from build123d import *

# Parameters (mm, degrees)
SKETCH1_R                    = 37.5
BOSS_EXTRUDE1_DEPTH          = 9.6
CUT_EXTRUDE2_START           = -9.6
CUT_EXTRUDE2_DEPTH           = 9.6
SKETCH4_R                    = 45
SKETCH4_R_2                  = 37.5
BOSS_EXTRUDE2_DEPTH          = 9.6
BOSS_EXTRUDE3_START          = -8.6
BOSS_EXTRUDE3_DEPTH          = 8.6
SKETCH7_R                    = 2
CUT_EXTRUDE3_DEPTH           = 65.359614666
SKETCH14_R                   = 5
SKETCH14_R_2                 = 2
BOSS_EXTRUDE5_DEPTH          = 1.5
CHAMFER1_SIZE                = 1.5
CIRPATTERN2_COUNT            = 3
CHAMFER1_OF_CIRPATTERN2_SIZE = 1.5
BOSS_EXTRUDE4_START          = -9.6
BOSS_EXTRUDE4_DEPTH          = 9.6
FILLET1_R                    = 10
SKETCH12_R                   = 1.5
CUT_EXTRUDE6_DEPTH           = 66.773550915
LPATTERN1_COUNT              = 10
LPATTERN1_PITCH              = 10
CUT_EXTRUDE7_DEPTH           = 66.773550915
FILLET3_R                    = 1
CIRPATTERN3_COUNT            = 3
FILLET3_OF_CIRPATTERN3_R     = 1


# Read off the part's stored shape, not the designer's step: Cut-Extrude2
# Some blends are built 0.0001 mm under size
with BuildPart() as part:
    # Sketch1 → Boss-Extrude1 (new body)
    with BuildSketch(Plane(origin=(0, 0, 0), x_dir=(1, 0, 0), z_dir=(0, 1, 0))):
        with Locations(Location((0, 0, 0), (0, 0, 270))):
            Circle(SKETCH1_R)
    extrude(amount=BOSS_EXTRUDE1_DEPTH)

    # Cut-Extrude2 outline → Cut-Extrude2 (cut)
    with BuildSketch(Plane(origin=(0, 9.6, 0), x_dir=(1, 0, 0), z_dir=(0, 1, 0)).offset(CUT_EXTRUDE2_START)):
        with BuildLine():
            ThreePointArc((-24.104535363, -28.726666617), (0, -24.760936498), (24.104535363, -28.726666617))
            ThreePointArc((24.104535363, -28.726666617), (32.475952642, -18.75), (36.930290738, -6.511806663))
            ThreePointArc((36.930290738, -6.511806663), (21.443600029, 12.380468249), (12.825755375, 35.238473279))
            ThreePointArc((12.825755375, 35.238473279), (0, 37.5), (-12.825755375, 35.238473279))
            ThreePointArc((-12.825755375, 35.238473279), (-21.443600029, 12.380468249), (-36.930290738, -6.511806663))
            ThreePointArc((-36.930290738, -6.511806663), (-32.475952642, -18.75), (-24.104535363, -28.726666617))
        make_face()
    extrude(amount=CUT_EXTRUDE2_DEPTH, mode=Mode.SUBTRACT)

    # Sketch4 → Boss-Extrude2 (add)
    with BuildSketch(Plane(origin=(0, 0, 0), x_dir=(1, 0, 0), z_dir=(0, 1, 0))):
        with Locations(Location((0, 0, 0), (0, 0, 270))):
            Circle(SKETCH4_R)
        Circle(SKETCH4_R_2, mode=Mode.SUBTRACT)
    extrude(amount=BOSS_EXTRUDE2_DEPTH)

    # Sketch6 → Boss-Extrude3 (add)
    with BuildSketch(Plane(origin=(0, 9.6, 0), x_dir=(1, 0, 0), z_dir=(0, 1, 0)).offset(BOSS_EXTRUDE3_START)):
        with BuildLine():
            ThreePointArc((24.104535363, -28.726666617), (32.475952642, -18.75), (36.930290738, -6.511806663))
            ThreePointArc((36.930290738, -6.511806663), (21.443600029, 12.380468249), (12.825755375, 35.238473279))
            ThreePointArc((12.825755375, 35.238473279), (0, 37.5), (-12.825755375, 35.238473279))
            ThreePointArc((-12.825755375, 35.238473279), (-21.443600029, 12.380468249), (-36.930290738, -6.511806663))
            ThreePointArc((-36.930290738, -6.511806663), (-32.475952642, -18.75), (-24.104535363, -28.726666617))
            ThreePointArc((-24.104535363, -28.726666617), (0, -24.760936498), (24.104535363, -28.726666617))
        make_face()
    extrude(amount=BOSS_EXTRUDE3_DEPTH)

    # Sketch7 → Cut-Extrude3 (cut, through all)
    with BuildSketch(Plane(origin=(0, 9.6, 0), x_dir=(1, 0, 0), z_dir=(0, 1, 0))):
        with Locations(Location((0, 18, 0), (0, 0, 270))):
            Circle(SKETCH7_R)
    cut_extrude3 = extrude(amount=-CUT_EXTRUDE3_DEPTH, mode=Mode.SUBTRACT)

    # Sketch14 → Boss-Extrude5 (add)
    with BuildSketch(Plane.XZ.offset(-1)):
        with Locations(Location((0, -18, 0), (0, 0, 90))):
            Circle(SKETCH14_R)
        with Locations(Location((0, -18, 0), (0, 0, 90))):
            Circle(SKETCH14_R_2, mode=Mode.SUBTRACT)
    boss_extrude5 = extrude(amount=BOSS_EXTRUDE5_DEPTH)

    # Chamfer1
    chamfer1_edges = [part.edges().sort_by_distance(p)[0] for p in [
        (0, 1, -23),
    ]]
    chamfer(chamfer1_edges, length=CHAMFER1_SIZE - 0.0001)  # a hair under: the kernel refuses the full size

    # CirPattern2: Cut-Extrude3, Boss-Extrude5 ×3 about axis
    cirpattern2_axis = Axis((0, 0, 0), (0, 1, 0))
    add([cut_extrude3.rotate(cirpattern2_axis, i * 360 / CIRPATTERN2_COUNT) for i in range(1, CIRPATTERN2_COUNT)], mode=Mode.SUBTRACT)
    add([boss_extrude5.rotate(cirpattern2_axis, i * 360 / CIRPATTERN2_COUNT) for i in range(1, CIRPATTERN2_COUNT)])

    # Chamfer1 of CirPattern2
    chamfer1_of_cirpattern2_edges = [part.edges().sort_by_distance(p)[0] for p in [
        (-19.918584287, 1, 11.5),
        (19.918584287, 1, 11.5),
    ]]
    chamfer(chamfer1_of_cirpattern2_edges, length=CHAMFER1_OF_CIRPATTERN2_SIZE - 0.0001)  # a hair under: the kernel refuses the full size

    # Sketch11 → Boss-Extrude4 (add)
    with BuildSketch(Plane(origin=(0, 9.6, 0), x_dir=(1, 0, 0), z_dir=(0, 1, 0)).offset(BOSS_EXTRUDE4_START)):
        with BuildLine():
            ThreePointArc((-22.449944321, 39), (0, 45), (22.449944321, 39))
            Line((22.449944321, 39), (25, 39))
            Line((25, 39), (25, 47))
            Line((25, 47), (-25, 47))
            Line((-25, 47), (-25, 39))
            Line((-25, 39), (-22.449944321, 39))
        make_face()
    extrude(amount=BOSS_EXTRUDE4_DEPTH)

    # Fillet1
    # the kernel refuses this fillet: 10 mm, written as the material it adds along each edge
    with BuildSketch(Plane(origin=(-22.449944321, 0, -39), x_dir=(-1, 0, 0), z_dir=(0, 1, 0))) as fillet1_piece_1:
        with BuildLine():
            CenterArc((11.645047875, -4.157056285), FILLET1_R, 128.309485754, 27.126753117)
            ThreePointArc((5.445958385, 3.689681222), (2.79048981, 1.745195143), (0, 0))
            Line((0, 0), (2.550055679, 0))
        make_face()
    extrude(amount=9.6)
    with BuildSketch(Plane(origin=(22.449944321, 0, -39), x_dir=(1, 0, 0), z_dir=(0, 1, 0))) as fillet1_piece_2:
        with BuildLine():
            CenterArc((11.645047875, 4.157056285), FILLET1_R, 204.563761129, 27.126753117)
            ThreePointArc((5.445958385, -3.689681222), (2.79048981, -1.745195143), (0, 0))
            Line((0, 0), (2.550055679, 0))
        make_face()
    extrude(amount=9.6)

    # Sketch12 → Cut-Extrude6 (cut, through all)
    with BuildSketch(Plane.XZ):
        with Locations(Location((-20, -43, 0), (0, 0, 270))):
            Circle(SKETCH12_R)
    cut_extrude6 = extrude(amount=-CUT_EXTRUDE6_DEPTH, mode=Mode.SUBTRACT)

    # LPattern1: Cut-Extrude6 ×10
    with Locations(*[(i * LPATTERN1_PITCH, 0, 0) for i in range(1, LPATTERN1_COUNT)]):
        add(cut_extrude6, mode=Mode.SUBTRACT)

    # Sketch13 → Cut-Extrude7 (cut, through all)
    with BuildSketch(Plane.XZ):
        with BuildLine():
            ThreePointArc((-22.11228446, 33.332369792), (0, 29.760936498), (22.11228446, 33.332369792))
            ThreePointArc((22.11228446, 33.332369792), (0, 40), (-22.11228446, 33.332369792))
        make_face()
    cut_extrude7 = extrude(amount=-CUT_EXTRUDE7_DEPTH, mode=Mode.SUBTRACT)

    # Fillet3
    fillet3_edges = [part.edges().sort_by_distance(p)[0] for p in [
        (-22.11228446, 4.8, 33.332369792),
        (22.11228446, 4.8, 33.332369792),
    ]]
    fillet(fillet3_edges, radius=FILLET3_R)

    # CirPattern3: Cut-Extrude7 ×3 about axis
    cirpattern3_axis = Axis((0, 0, 0), (0, 1, 0))
    for i in range(1, CIRPATTERN3_COUNT):
        add(cut_extrude7.rotate(cirpattern3_axis, i * 360 / CIRPATTERN3_COUNT), mode=Mode.SUBTRACT)

    # Fillet3 of CirPattern3
    fillet3_of_cirpattern3_edges = [part.edges().sort_by_distance(p)[0] for p in [
        (39.922821238, 4.8, 2.483615182),
        (17.810536778, 4.8, -35.815984974),
        (-17.810536778, 4.8, -35.815984974),
        (-39.922821238, 4.8, 2.483615182),
    ]]
    fillet(fillet3_of_cirpattern3_edges, radius=FILLET3_OF_CIRPATTERN3_R)


solid = part.part
Design review of the part built by this model. Coordinates are the model's own, in mm. A direction names the side the tool comes from. Coordinates: 2 decimals unless noted, no trailing zeros. Order: outer loops, then holes, each group sorted by start corner. A loop starts at its lowest first (then second) coordinate and runs counter-clockwise, first axis right, second up. Notation, with made-up numbers: M -2.5,72 L 50.5,72 A15 cw 50.5,94 Z; hole C 10.25,-20.5 d8. An arc over 180 degrees is marked long. Use a Markdown table: item, result.
(1) For P1, Ø2, axis at y = 2, z = -23, coming from the +X side; P2, Ø2, axis at y = 6.5, z = 3.5, coming from the -X side; P3, Ø5, axis at x = 14.5, y = 2.5, coming from the +Z side, all flat-tipped, find the tip position at first contact; note any pin that passes through.
Worked answers:
| item | result |
|---|---|
| P1 | stops at x = 39.26 |
| P2 | stops at x = -44.93 |
| P3 | stops at z = 43.37 |
(2) For faces 1 (the cylindrical face through (32.384, 0.493, 18.908)), 2 (the cylindrical face through (-25.63, 4.73, -15.13)), 3 (the flat face through (2.2, -0.5, -18.1)), list the 3-axis set-ups (+Z, -Z, +X, -X, +Y, -Y) from which the entire face can be reached by the end or side of a thin tool; tool diameter is ignored.
Worked answers:
| item | result |
|---|---|
| face 1 | -Y |
| face 2 | +Y, -Y |
| face 3 | +Z, -Z, +X, -X, -Y |
(3) Add section C-C (z = 17.5). Give the boundary of the cut face in (x, y), then the cut area to 3 significant figures.
Worked answers:
| item | result |
|---|---|
| outline | M -41.46,0 L -33.17,0 L -33.17,1 L 33.17,1 L 33.17,0 L 41.46,0 L 41.46,9.6 L -41.46,9.6 Z |
| area | 730 mm2 |
(4) Wall thickness on probe 1 along X at (y, z) = (7.25, -43); probe 2 along Z at (x, y) = (-9, 0.5); probe 3 along X at (y, z) = (0.75, 7.5): over which ranges is each line inside the solid? List them lowest first.
Worked answers:
| item | result |
|---|---|
| probe 1 | x = -25 to -21.5, -18.5 to -11.5, -8.5 to -1.5, 1.5 to 8.5, 11.5 to 18.5, 21.5 to 25 |
| probe 2 | z = -47 to -44.12, -41.88 to -36.4, 25.3 to 30.34, 38.97 to 44.09 |
| probe 3 | x = -44.37 to -36.74, -21.66 to -16.91, -14.27 to -9.52, 9.52 to 14.27, 16.91 to 21.66, 36.74 to 44.37 |
(5) Add section A-A (x = -34). Give the boundary of the cut face in (y, z), then the cut area to 3 significant figures.
Worked answers:
| item | result |
|---|---|
| outline | M 0,-29.48 L 9.6,-29.48 L 9.6,-21.07 L 0,-21.07 Z; M 0,-3.45 L 9.6,-3.45 L 9.6,29.48 L 0,29.48 L 0,15.82 L 1,15.82 L 1,3.79 L 0,3.79 Z |
| area | 385 mm2 |
(6) Add section B-B (z = -2). Give the boundary of the cut face in (x, y), then the cut area to 3 significant figures.
Worked answers:
| item | result |
|---|---|
| outline | M -44.96,0 L -39.95,0 L -39.95,9.6 L -44.96,9.6 Z; M -35.32,0 L -28.66,0 L -28.66,1 L 28.66,1 L 28.66,0 L 35.32,0 L 35.32,9.6 L -35.32,9.6 Z; M 39.95,0 L 44.96,0 L 44.96,9.6 L 39.95,9.6 Z |
| area | 717 mm2 |
(7) Add section D-D (y = 4.25). Count the separate pieces of the cut face and the enclosed holes in it, then the cut area to 3 significant figures.
Worked answers:
| item | result |
|---|---|
| separate pieces | 1 |
| enclosed holes | 11 |
| area | 5,600 mm2 |
